Geometry check sheet. Reference: the model listing, model coordinates, mm. A direction names the side the tool comes from. Give positions to 0.01 mm unless a question says otherwise; leave off trailing zeros. Write each loop counter-clockwise with the first axis right and the second up, starting at its lowest first coordinate (ties: lowest second). Pieces come first, ordered by that corner, then holes. Notation, with made-up numbers: (88, 19.25) -> (103, 19.25) arc R13 cw to (103, 39.25) -> close; hole circle Ø5 at (49, 59). An arc over 180 degrees is marked (long way). Write item = value, one per line. Start each with the question number.
1. Cross-section at B-B, the plane y = -3.8. Record the cut outline in (x, z), plus the area to 3 significant figures.
2. Set-up check for faces 1 (the flat face through (0, -4, -11)), 2 (the flat face through (0, -4, 11)), 3 (the flat face through (0, -3, 0)): record each of +Z, -Z, +X, -X, +Y, -Y from which the full face is reachable in a straight line by a thin tool's end or side.
3. Cross-section at C-C, the plane z = 4. Record the cut outline in (x, y).
4. Cross-section at A-A, the plane x = 0. Record the cut outline in (y, z), plus the area to 3 significant figures.
5. Cross-section at D-D, the plane x = -9.5. Record the cut outline in (y, z).
6. Depth check by flat-ended pin: P1, Ø8, axis at x = 7.5, z = 6.5, coming from the +Y side; P2, Ø6, axis at x = 0, z = 0, coming from the -Y side; P3, Ø1, axis at y = -4, z = -8.5, coming from the -X side. Enter the tip coordinate at first touch or a pass-through.
7. Thickness scan on line 1 along Z through (x, y) = (0, -4.35); line 2 along X through (y, z) = (-3.45, -5.25); line 3 along Z through (x, y) = (-9, -4.7). Record the ranges inside material, lowest first.
```python
from build123d import *

# Parameters (mm, degrees)
F0_W     = 37
F0_H     = 24
F1_DEPTH = 2.5
F2_W     = 35
F2_H     = 22
F3_DEPTH = 2.5
F4_R     = 5
F5_DEPTH = 2


with BuildPart() as f1:
    # F0 (on Front) → F1 (new body)
    with BuildSketch(Plane.XZ):
        Rectangle(F0_W, F0_H)
    extrude(amount=F1_DEPTH)

    # F2 (on face) → F3 (join)
    with BuildSketch(Plane.XZ.offset(2.5)):
        Rectangle(F2_W, F2_H)
    extrude(amount=F3_DEPTH)

    # F4 (on face) → F5 (cut)
    with BuildSketch(Plane.XZ.offset(5)):
        Circle(F4_R)
    extrude(amount=-F5_DEPTH, mode=Mode.SUBTRACT)


solid = f1.part
```
Answers:
q1.outline = (-17.5, -11) -> (17.5, -11) -> (17.5, 11) -> (-17.5, 11) -> close; hole circle Ø10 at (0, 0)
q1.area = 691 mm^2
q2.face_1 = -Z, +X, -X, -Y
q2.face_2 = +Z, +X, -X, -Y
q2.face_3 = -Y
q3.outline = (-18.5, -2.5) -> (-17.5, -2.5) -> (-17.5, -5) -> (-3, -5) -> (-3, -3) -> (3, -3) -> (3, -5) -> (17.5, -5) -> (17.5, -2.5) -> (18.5, -2.5) -> (18.5, 0) -> (-18.5, 0) -> close
q4.outline = (-5, -11) -> (-2.5, -11) -> (-2.5, -12) -> (0, -12) -> (0, 12) -> (-2.5, 12) -> (-2.5, 11) -> (-5, 11) -> (-5, 5) -> (-3, 5) -> (-3, -5) -> (-5, -5) -> close
q4.area = 95.0 mm^2
q5.outline = (-5, -11) -> (-2.5, -11) -> (-2.5, -12) -> (0, -12) -> (0, 12) -> (-2.5, 12) -> (-2.5, 11) -> (-5, 11) -> close
q6.P1 = 0
q6.P2 = -3
q6.P3 = -17.5
q7.line_1 = -11 to -5, 5 to 11
q7.line_2 = -17.5 to 17.5
q7.line_3 = -11 to 11
